from build123d import *

# Parameters (mm, degrees)
F0_W     = 101.6
F0_H     = 12.7
F1_DEPTH = 12.7
F0_H_2   = 31.75
F2_DEPTH = 6.35
F3_W     = 152.4
F3_H     = 19.05
F4_DEPTH = 6.35
F5_W     = 76.2
F5_H     = 19.05
F6_DEPTH = 10.16
F7_R     = 5.08


with BuildPart() as f1:
    # F0 (on Front) → F1 (new body, symmetric)
    with BuildSketch(Plane.XZ):
        with BuildLine():
            Line((-50.8, 19.05), (-50.8, 31.75))
            ThreePointArc((-50.8, 31.75), (-69.3027203169, 26.6045338614), (-82.55, 12.7))
            Line((-82.55, 12.7), (-82.55, -31.75))
            Line((-82.55, -31.75), (-50.8, -31.75))
            Line((-50.8, -31.75), (-50.8, -12.7))
            Line((-50.8, -12.7), (-50.8, 19.05))
        make_face()
        with Locations((0, 25.4)):
            Rectangle(F0_W, F0_H)
        with BuildLine():
            Line((54.74242965, 31.75), (50.8, 31.75))
            Line((50.8, 31.75), (50.8, 19.05))
            Line((50.8, 19.05), (50.8, -12.7))
            Line((50.8, -12.7), (-50.8, -12.7))
            Line((-50.8, -12.7), (-50.8, -31.75))
            Line((-50.8, -31.75), (82.55, -31.75))
            Line((82.55, -31.75), (82.55, 12.7))
            ThreePointArc((82.55, 12.7), (71.2844870911, 26.0761255456), (54.74242965, 31.75))
        make_face()
    extrude(amount=F1_DEPTH, both=True)

    # F0 (on Front) → F2 (join, symmetric)
    with BuildSketch(Plane.XZ):
        with Locations((0, 3.175)):
            Rectangle(F0_W, F0_H_2)
    extrude(amount=F2_DEPTH, both=True)

    # F3 (on face) → F4 (cut)
    with BuildSketch(Plane(origin=(0, 0, -31.75), x_dir=(1, 0, 0), z_dir=(0, 0, -1))):
        Rectangle(F3_W, F3_H)
    extrude(amount=-F4_DEPTH, mode=Mode.SUBTRACT)

    # F5 (on face) → F6 (cut)
    with BuildSketch(Plane(origin=(0, 0, -25.4), x_dir=(1, 0, 0), z_dir=(0, 0, -1))):
        Rectangle(F5_W, F5_H)
    extrude(amount=-F6_DEPTH, mode=Mode.SUBTRACT)

    # F7
    f7_edges = [f1.edges().sort_by_distance(p)[0] for p in [
        (-38.1, -9.525, -20.32),
        (38.1, -9.525, -20.32),
        (38.1, 9.525, -20.32),
        (-38.1, 9.525, -20.32),
        (-50.8, -9.525, 19.05),
        (-50.8, -9.525, -12.7),
        (50.8, -9.525, 19.05),
        (50.8, -9.525, -12.7),
        (50.8, 9.525, 19.05),
        (50.8, 9.525, -12.7),
        (-50.8, 9.525, 19.05),
        (-50.8, 9.525, -12.7),
    ]]
    fillet(f7_edges, radius=F7_R)


solid = f1.part
CAD build for the part. Positions are in the model's coordinates, mm. A direction names the side the tool comes from. Round coordinates to 2 decimals unless told otherwise and drop trailing zeros. Order: outer loops, then holes, each group sorted by start corner. A loop starts at its lowest first (then second) coordinate and runs counter-clockwise, first axis right, second up. Notation, with made-up numbers: (88, 38) - (111, 38) arc R18 cw to (111, 48) - close; hole circle Ø5 at (-16.5, 43). An arc over 180 degrees is marked (long way). Return JSON: item names as keys, results as strings.
(1) Cut at B-B (y = -0.75). Give the cut face in (x, z), then the cut area to 3 significant figures.
Answer key:
{"outline": "(-82.55, -31.75) - (-76.2, -31.75) - (-76.2, -25.4) - (-38.1, -25.4) - (-38.1, -15.24) - (38.1, -15.24) - (38.1, -25.4) - (76.2, -25.4) - (76.2, -31.75) - (82.55, -31.75) - (82.55, 12.7) arc R32.76 ccw to (54.74, 31.75) - (-50.8, 31.75) arc R36.11 ccw to (-82.55, 12.7) - close", "area": "8,410 mm^2"}
(2) Pin check, flat tips, straight feed: pin 1 Ø1.5 at (y, z) = (-1, 20) entering from -X; pin 2 Ø8 at (x, y) = (56, 1) entering from -Z; pin 3 Ø16 at (x, z) = (-12, -0.5) entering from -Y. Stop position of each tip, or through.
Answer key:
{"pin 1": "stops at x = -78.05", "pin 2": "stops at z = -25.4", "pin 3": "stops at y = -6.35"}
(3) Tool access for faces 1 (the face through (-49.351, 9.569, -11.172)), 2 (the face through (-36.57, -8.08, -20.25)), 3 (the face through (1, -10, -12.7)): list every direction of +Z, -Z, +X, -X, +Y, -Y with a clear straight run to the whole face (end or side of a thin tool).
Answer key:
{"face 1": "+Y", "face 2": "-Z", "face 3": "-Y"}
(4) Cut at A-A (z = 9). Give the cut face in (x, y).
Answer key:
{"outline": "(-82.55, -12.7) - (-50.8, -12.7) - (-50.8, -6.35) - (50.8, -6.35) - (50.8, -12.7) - (82.55, -12.7) - (82.55, 12.7) - (50.8, 12.7) - (50.8, 6.35) - (-50.8, 6.35) - (-50.8, 12.7) - (-82.55, 12.7) - close"}
(5) Cut at D-D (y = 8). Give the cut face in (x, z).
Answer key:
{"outline": "(-82.55, -31.75) - (-76.2, -31.75) - (-76.2, -25.4) - (-36.65, -25.4) - (-36.65, -15.24) - (36.65, -15.24) - (36.65, -25.4) - (76.2, -25.4) - (76.2, -31.75) - (82.55, -31.75) - (82.55, 12.7) arc R32.76 ccw to (54.74, 31.75) - (-50.8, 31.75) arc R36.11 ccw to (-82.55, 12.7) - close; hole (-50.8, -7.62) arc R5.08 ccw to (-45.72, -12.7) - (45.72, -12.7) arc R5.08 ccw to (50.8, -7.62) - (50.8, 13.97) arc R5.08 ccw to (45.72, 19.05) - (-45.72, 19.05) arc R5.08 ccw to (-50.8, 13.97) - close"}
(6) Wall check: probe 1 along X at (y, z) = (-9.75, -8); probe 2 along X at (y, z) = (0.75, -21); probe 3 along Y at (x, z) = (8.5, -21) (3 decimals). Give the ranges that are in metal, low to high. Write a range as from..to.
Answer key:
{"probe 1": "x = -82.55..-50.79, 50.79..82.55", "probe 2": "x = -82.55..-38.1, 38.1..82.55", "probe 3": "y = -12.7..-9.525, 9.525..12.7"}
(7) Pull direction X, two halves, no side cores. Call faces 4 (the face through (-1, 12.7, -14)), 5 (the face through (50.8, 9, 3)), 6 (the face through (-69.069, -0.178, 26.744)): +X half, -X half, draft (parallel to the pull), parting line (faces both ways), or undercut.
Answer key:
{"face 4": "draft", "face 5": "undercut", "face 6": "-X half"}
(8) Cut at C-C (x = 22). Give the cut face in (y, z) (3 decimals), then the cut area to 3 significant figures.
Answer key:
{"outline": "(-12.7, -31.75) - (-9.525, -31.75) - (-9.525, -15.24) - (9.525, -15.24) - (9.525, -31.75) - (12.7, -31.75) - (12.7, -12.7) - (6.35, -12.7) - (6.35, 19.05) - (12.7, 19.05) - (12.7, 31.75) - (-12.7, 31.75) - (-12.7, 19.05) - (-6.35, 19.05) - (-6.35, -12.7) - (-12.7, -12.7) - close", "area": "895 mm^2"}
